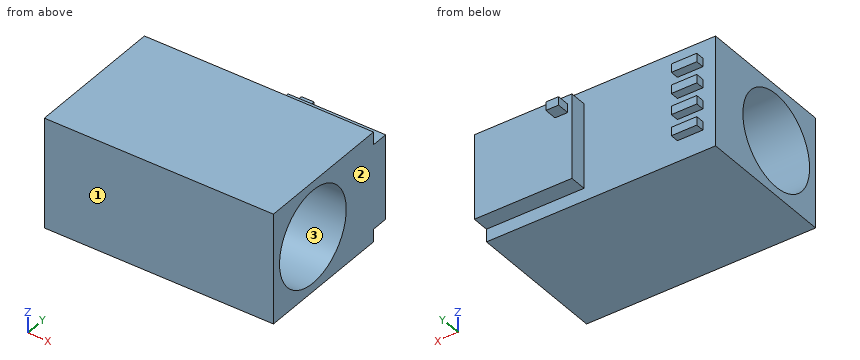
```python
from build123d import *

# Parameters (mm, degrees)
DODANIE_WYCI_GNI_CIE1_DEPTH = 130
SZKIC2_W                    = 115
SZKIC2_H                    = 15
WYTNIJ_WYCI_GNI_CIE1_DEPTH  = 20
SZKIC3_W                    = 30
SZKIC3_H                    = 10
DODANIE_WYCI_GNI_CIE2_DEPTH = 10
SZKIC4_W                    = 15
SZKIC4_H                    = 10
DODANIE_WYCI_GNI_CIE3_DEPTH = 15
SZKIC5_R                    = 55
WYTNIJ_WYCI_GNI_CIE2_DEPTH  = 361.277670693


with BuildPart() as part:
    # Szkic1 → Dodanie-wyciągnięcie1 (new body)
    with BuildSketch(Plane.XY):
        Polygon((135, 0), (-135, 0), (-135, 165), (20, 165), (20, 185), (135, 185), align=None)
    extrude(amount=DODANIE_WYCI_GNI_CIE1_DEPTH)

    # Szkic2 → Wytnij-wyciągnięcie1 (cut)
    with BuildSketch(Plane(origin=(0, 185, 0), x_dir=(1, 0, 0), z_dir=(0, 1, 0))):
        with Locations((77.5, -122.5)):
            Rectangle(SZKIC2_W, SZKIC2_H)
        with Locations((77.5, -7.5)):
            Rectangle(SZKIC2_W, SZKIC2_H)
    extrude(amount=-WYTNIJ_WYCI_GNI_CIE1_DEPTH, mode=Mode.SUBTRACT)

    # Szkic3 → Dodanie-wyciągnięcie2 (add)
    with BuildSketch(Plane(origin=(0, 165, 0), x_dir=(1, 0, 0), z_dir=(0, 1, 0))):
        with Locations((-105, -105)):
            Rectangle(SZKIC3_W, SZKIC3_H)
        with Locations((-105, -80)):
            Rectangle(SZKIC3_W, SZKIC3_H)
        with Locations((-105, -55)):
            Rectangle(SZKIC3_W, SZKIC3_H)
        with Locations((-105, -30)):
            Rectangle(SZKIC3_W, SZKIC3_H)
    extrude(amount=DODANIE_WYCI_GNI_CIE2_DEPTH)

    # Szkic4 → Dodanie-wyciągnięcie3 (add)
    with BuildSketch(Plane(origin=(0, 185, 0), x_dir=(1, 0, 0), z_dir=(0, 1, 0))):
        with Locations((32.5, -100)):
            Rectangle(SZKIC4_W, SZKIC4_H)
    extrude(amount=DODANIE_WYCI_GNI_CIE3_DEPTH)

    # Szkic5 → Wytnij-wyciągnięcie2 (cut, through all)
    with BuildSketch(Plane.ZY.offset(135)):
        with Locations((65, 65)):
            Circle(SZKIC5_R)
    extrude(amount=-WYTNIJ_WYCI_GNI_CIE2_DEPTH, mode=Mode.SUBTRACT)


solid = part.part
```
Verification items for the finished model (mm, model axes). Face numbers are marked on the shaded views. Give positions to 0.01 mm unless a question says otherwise; leave off trailing zeros. Write each loop counter-clockwise with the first axis right and the second up, starting at its lowest first coordinate (ties: lowest second). Pieces come first, ordered by that corner, then holes. Notation, with made-up numbers: M 55,30.25 L 96,30.25 A13 cw 96,50.25 Z; hole C 29.5,80.25 d5. An arc over 180 degrees is marked long. One line per question, with ' | ' between items.
1) Section check A-A on z = 65. Enter the section's corners in (x, y).
Result:
outline: M -135,0 L 135,0 L 135,10 L -135,10 Z; M -135,120 L 135,120 L 135,185 L 20,185 L 20,165 L -135,165 Z
2) Thickness scan on line 1 along Z through (x, y) = (123.5, 177); line 2 along Y through (x, z) = (66, 65); line 3 along Y through (x, z) = (112, 7). Record the ranges inside material, lowest first. Write a range as [from, to].
Result:
line 1: z = [15, 115] | line 2: y = [0, 10], [120, 185] | line 3: y = [0, 165]
3) Mould release check, pull along Y, two halves, no side actions. Record for the marked faces 1, 2 and 3: released by +Y, released by -Y, zero draft, split by the parting line, or undercut.
Result:
face 1: released by -Y | face 2: zero draft | face 3: undercut
4) Gauge pin test, flat ends, axial feed: pin 1 Ø3 at (x, z) = (-107, 56.5) entering from +Y; pin 2 Ø7.5 at (x, y) = (34.5, 189.5) entering from -Z; pin 3 Ø3 at (y, z) = (170.5, 54.5) entering from -X. Record the tip position at first contact, or that the pin passes through.
Result:
pin 1: stops at y = 175 | pin 2: stops at z = 95 | pin 3: stops at x = -120
5) Section check D-D on x = -96. Enter the section's corners in (y, z), plus the area to 3 significant figures.
Result:
outline: M 0,0 L 165,0 L 165,25 L 175,25 L 175,35 L 165,35 L 165,50 L 175,50 L 175,60 L 165,60 L 165,75 L 175,75 L 175,85 L 165,85 L 165,100 L 175,100 L 175,110 L 165,110 L 165,130 L 0,130 Z; hole C 65,65 d110 | area: 12,300 mm2
6) Section check C-C on y = 65. Enter the section's corners in (x, z).
Result:
outline: M -135,0 L 135,0 L 135,10 L -135,10 Z; M -135,120 L 135,120 L 135,130 L -135,130 Z
7) Section check B-B on x = 35.5. Enter the section's corners in (y, z), plus the area to 3 significant figures.
Result:
outline: M 0,0 L 165,0 L 165,15 L 185,15 L 185,95 L 200,95 L 200,105 L 185,105 L 185,115 L 165,115 L 165,130 L 0,130 Z; hole C 65,65 d110 | area: 14,100 mm2
